Print and shaded views of the part. All mm, measured from the part's lowest x, y and z. A direction names the side the tool comes from. Coordinates: 2 decimals unless noted, no trailing zeros. Write each loop counter-clockwise with the first axis right and the second up, starting at its lowest first coordinate (ties: lowest second). Pieces come first, ordered by that corner, then holes. Notation, with made-up numbers: (47.5, 82) -> (91.5, 82) arc R8 cw to (91.5, 90) -> close; hole circle Ø9 at (22.25, -11). An arc over 180 degrees is marked (long way). Write item = value, one per line.
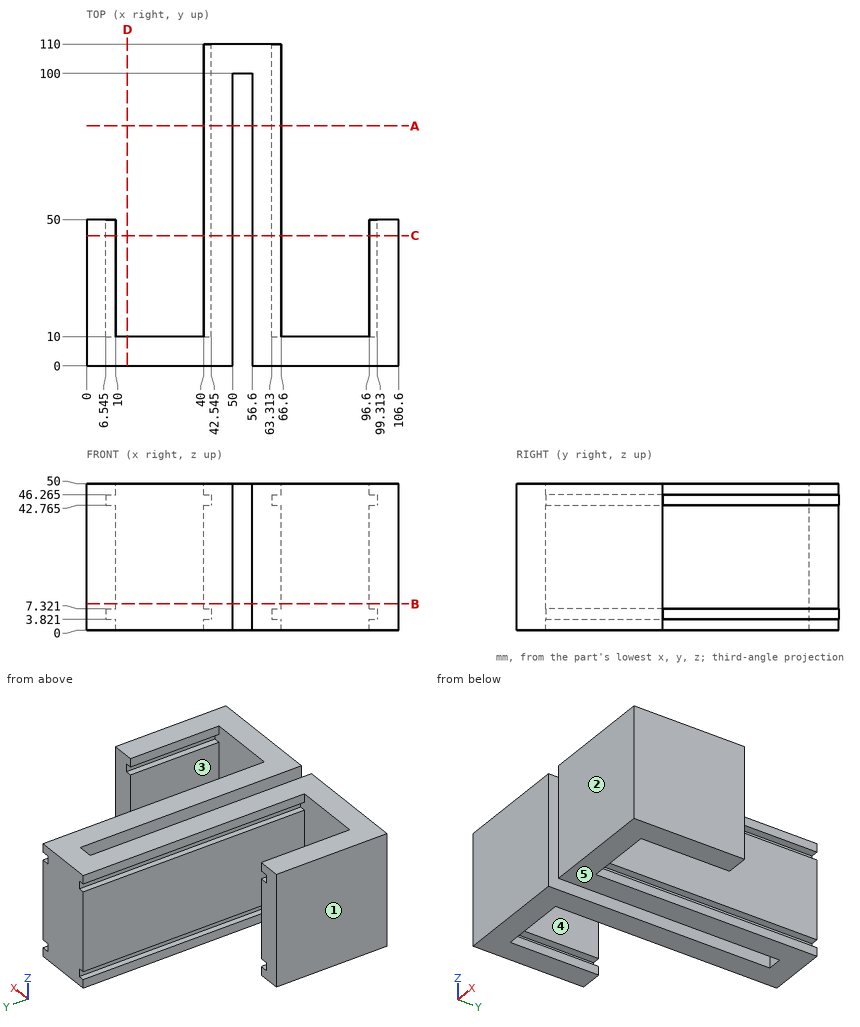
Q1. Saw through at B-B on z = 9. Give the cut face in (x, y), and give its area (3 significant figures).
Model answer:
outline = (0, 0) -> (50, 0) -> (50, 100) -> (56.6, 100) -> (56.6, 0) -> (106.6, 0) -> (106.6, 50) -> (96.6, 50) -> (96.6, 10) -> (66.6, 10) -> (66.6, 110) -> (40, 110) -> (40, 10) -> (10, 10) -> (10, 50) -> (0, 50) -> close
area = 3,870 mm²
Q2. Which spindle directions (+Z, -Z, +X, -X, +Y, -Y) get a long thin tool onto all of the face, cutting with end or side? Do the marked faces 4 and 5. Say none if no direction does.
Model answer:
face_4 = +Z, -Z, +Y
face_5 = -Z, +X, -X, +Y, -Y
Q3. Mould opens along X. For the marked faces 1, 2 and 3 say: released by +X, released by -X, zero draft, split by the parting line, or undercut.
Model answer:
face_1 = released by -X
face_2 = zero draft
face_3 = undercut
Q4. Pin check, flat tips, straight feed: pin 1 (5.5 mm diameter, centred on x = 53.5, z = 17, fed in from -Y); pin 2 (1 mm diameter, centred on y = 79, z = 6.5, fed in from -X) (3 decimals); pin 3 (11 mm diameter, centred on x = 30, z = 26.5, fed in from +Y). Stop position of each tip, or through.
Model answer:
pin_1 = 100
pin_2 = 42.545
pin_3 = 10
Q5. Saw through at D-D on x = 14. Give the cut face in (y, z).
Model answer:
outline = (0, 0) -> (10, 0) -> (10, 50) -> (0, 50) -> close
Q6. Saw through at A-A on y = 82. Give the cut face in (x, z) (1 decimal), and give its area (3 significant figures).
Model answer:
outline = (40, 0) -> (50, 0) -> (50, 50) -> (40, 50) -> (40, 46.3) -> (42.5, 46.3) -> (42.5, 42.8) -> (40, 42.8) -> (40, 7.3) -> (42.5, 7.3) -> (42.5, 3.8) -> (40, 3.8) -> close; (56.6, 0) -> (66.6, 0) -> (66.6, 3.8) -> (63.3, 3.8) -> (63.3, 7.3) -> (66.6, 7.3) -> (66.6, 42.8) -> (63.3, 42.8) -> (63.3, 46.3) -> (66.6, 46.3) -> (66.6, 50) -> (56.6, 50) -> close
area = 959 mm²
Q7. Probe line 1 (X direction, y = 13, z = 20.5); line 2 (X direction, y = 47, z = 6) (1 decimal); line 3 (Z direction, x = 63.5, y = 60.5) (1 decimal). List the from-to ranges inside material, lowest first. Write a range as from..to.
Model answer:
line_1 = 0..10, 40..50, 56.6..66.6, 96.6..106.6
line_2 = 0..6.5, 42.5..50, 56.6..63.3, 99.3..106.6
line_3 = 0..3.8, 7.3..42.8, 46.3..50
Q8. Saw through at C-C on y = 44.5. Count the separate pieces of the cut face and the enclosed holes in it, and give its area (3 significant figures).
Model answer:
separate_pieces = 4
enclosed_holes = 0
area = 1,920 mm²
